The listing builds one solid part. Answer for the finished solid, in the listing's coordinates (mm). A direction names the side the tool comes from. Round coordinates to 2 decimals unless told otherwise and drop trailing zeros. Loops run counter-clockwise (first coordinate to the right, second up) from the corner with the lowest first, then second, coordinate; pieces in that order, holes last. Notation, with made-up numbers: (63, -19) - (122, -19) arc R21 cw to (122, -6) - close; hole circle Ø4 at (30, 65). An arc over 180 degrees is marked (long way). One line per item, written item: value.
```python
from build123d import *

# Parameters (mm, degrees)
RESSALTO_EXTRUS_O1_DEPTH = 153
CASCA1_T                 = -3
CORTE_EXTRUS_O1_REACH    = 299.454
ESBO_O4_W                = 123
ESBO_O4_H                = 100
ESBO_O5_R                = 2
CORTE_EXTRUS_O2_DEPTH    = 154
ESBO_O6_R                = 2
CORTE_EXTRUS_O3_DEPTH    = 233.16


with BuildPart() as part:
    # Esboço1 → Ressalto-extrusão1 (new body)
    with BuildSketch(Plane.XY):
        with BuildLine():
            Line((0, 0), (0, 50))
            ThreePointArc((0, 50), (4.650495405, 69.922787932), (17.640776843, 85.72776103))
            Line((17.640776843, 85.72776103), (297.45381486, 300))
            Line((297.45381486, 300), (297.45381486, 150))
            Line((297.45381486, 150), (232.16, 100))
            Line((232.16, 100), (232.16, 0))
            Line((232.16, 0), (0, 0))
        make_face()
    extrude(amount=RESSALTO_EXTRUS_O1_DEPTH)

    # Casca1
    casca1_openings = [part.faces().sort_by_distance(p)[0] for p in [
        (116.08, 0, 76.5),
    ]]
    offset(amount=CASCA1_T, openings=casca1_openings, kind=Kind.INTERSECTION)

    # Esboço4 → Corte-extrusão1 (cut, up to next)
    with BuildSketch(Plane(origin=(297.45381486, 0, 0), x_dir=(0, 0, -1), z_dir=(1, 0, 0)), mode=Mode.PRIVATE) as corte_extrus_o1_sk1:
        with Locations((-76.5, 230)):
            Rectangle(ESBO_O4_W, ESBO_O4_H)
    corte_extrus_o1_tool1 = extrude(corte_extrus_o1_sk1.sketch, amount=-CORTE_EXTRUS_O1_REACH, mode=Mode.PRIVATE) & part.part
    add(corte_extrus_o1_tool1.solids().sort_by_distance((297.453815, 230, 76.5))[0], mode=Mode.SUBTRACT)

    # Esboço5 → Corte-extrusão2 (cut, through all)
    with BuildSketch(Plane.XY.offset(153)):
        with Locations((181.08, 5)):
            Circle(ESBO_O5_R)
        with Locations((51.08, 5)):
            Circle(ESBO_O5_R)
    extrude(amount=-CORTE_EXTRUS_O2_DEPTH, mode=Mode.SUBTRACT)

    # Esboço6 → Corte-extrusão3 (cut, through all)
    with BuildSketch(Plane(origin=(232.16, 0, 0), x_dir=(0, 0, -1), z_dir=(1, 0, 0))):
        with Locations((-36.5, 5)):
            Circle(ESBO_O6_R)
        with Locations((-116.5, 5)):
            Circle(ESBO_O6_R)
    extrude(amount=-CORTE_EXTRUS_O3_DEPTH, mode=Mode.SUBTRACT)


solid = part.part
```
1) A cutting plane is placed at A-A on z = 44.5. Give the vertices of the cut face in (x, y), and give its area (3 significant figures).
Final values:
outline: (0, 0) - (3, 0) - (3, 50) arc R42 cw to (19.46, 83.35) - (294.45, 293.92) - (294.45, 280) - (297.45, 280) - (297.45, 300) - (17.64, 85.73) arc R45 ccw to (0, 50) - close; (229.16, 0) - (232.16, 0) - (232.16, 100) - (297.45, 150) - (297.45, 180) - (294.45, 180) - (294.45, 151.48) - (229.16, 101.48) - close
area: 2,010 mm2
2) For a pull along Z with two mould halves and no side action, classify faces 1 (the flat face through (151, 116, 3)), 2 (the flat face through (151, 119, 0)), 3 (the flat face through (232.16, 51, 75)) as released by +Z, released by -Z, zero draft, split by the parting line, or undercut.
Final values:
face 1: undercut
face 2: released by -Z
face 3: zero draft
3) A cutting plane is placed at B-B on y = 40. Give the vertices of the cut face in (x, z).
Final values:
outline: (0, 0) - (232.16, 0) - (232.16, 153) - (0, 153) - close; hole (3, 3) - (229.16, 3) - (229.16, 150) - (3, 150) - close
4) Each of these flat-tipped pins is pushed along its axis until it touches: pin 1 Ø3 at (y, z) = (5, 36.5) entering from -X; pin 2 Ø1 at (y, z) = (157.5, 124.5) entering from -X; pin 3 Ø3 at (x, z) = (72.5, 56) entering from -Y; pin 4 Ø25 at (y, z) = (31, 88.5) entering from +X. Where does it stop, or does it pass through?
Final values:
pin 1: through
pin 2: x = 110.71
pin 3: y = 122.81
pin 4: x = 232.16
5) For faces 4 (the flat face through (3, 25, 75)), 5 (the flat face through (297.454, 176, 75)), 6 (the flat face through (294.454, 176, 75)), determine the directions among +Z, -Z, +X, -X, +Y, -Y from which every point of the face is accessible in a straight line to the end or side of a thin tool.
Final values:
face 4: -Y
face 5: +Z, -Z, +X, +Y, -Y
face 6: none
6) A cutting plane is placed at C-C on x = 59. Give the vertices of the cut face in (y, z), and give its area (3 significant figures).
Final values:
outline: (0, 0) - (117.4, 0) - (117.4, 153) - (0, 153) - (0, 150) - (113.62, 150) - (113.62, 3) - (0, 3) - close
area: 1,260 mm2
7) A cutting plane is placed at D-D on y = 261.5. Give the vertices of the cut face in (x, z).
Final values:
outline: (247.18, 0) - (297.45, 0) - (297.45, 15) - (294.45, 15) - (294.45, 3) - (252.11, 3) - (252.11, 150) - (294.45, 150) - (294.45, 138) - (297.45, 138) - (297.45, 153) - (247.18, 153) - close
8) Consider L1, parallel to Z at x = 157, y = 178; L2, parallel to Y at x = 230, z = 116; L3, parallel to X at y = 151, z = 33. Determine where each line is inside the solid, lowest interval first.
Final values:
L1: 0 to 3, 150 to 153
L2: 0 to 3.06, 6.94 to 102.12, 244.57 to 248.35
L3: 102.88 to 107.81, 293.83 to 297.45
